from build123d import *

# Parameters (mm, degrees)
SKIZZE4_R                                   = 11.5
SCHNITT_LINEAR_AUSTRAGEN1_DEPTH             = 2.1
SCHNITT_LINEAR_START                        = -8
SKIZZE5_R                                   = 1
SCHNITT_LINEAR_AUSTRAGEN2_DEPTH             = 1
SCHNITT_LINEAR_AUSTRAGEN3_REACH             = 31.825
SCHNITT_LINEAR_AUSTRAGEN3_DIRECTION_2_DEPTH = 18.575
SKIZZE7_R                                   = 0.85
SCHNITT_LINEAR_AUSTRAGEN4_DEPTH             = 10


with BuildPart() as part:
    # Skizze3 → Rotation1 (revolve)
    with BuildSketch(Plane(origin=(0, 0, 0), x_dir=(0, 0, -1), z_dir=(1, 0, 0))):
        Polygon((-1.5, 4.2), (0, 4.2), (0, 0.5), (11, 0.5), (11, 4.2), (12.5, 4.2), (12.5, -12.875), (-1.5, -12.875), align=None)
    revolve(axis=Axis((0, -19.5, -13), (0, 0, 1)))

    # Skizze4 → Schnitt-Linear austragen1 (cut)
    with BuildSketch(Plane.XY.offset(1.5)):
        with Locations((0, -19.5)):
            Circle(SKIZZE4_R)
    extrude(amount=-SCHNITT_LINEAR_AUSTRAGEN1_DEPTH, mode=Mode.SUBTRACT)

    # Skizze5 → Schnitt-Linear austragen2 (cut)
    with BuildSketch(Plane.XY.offset(1.5).offset(SCHNITT_LINEAR_START)):
        with Locations((6.01040764, -13.48959236)):
            Circle(SKIZZE5_R)
        with Locations((7.573555456, -23.358919248)):
            Circle(SKIZZE5_R)
        with Locations((-1.329692953, -27.895350895)):
            Circle(SKIZZE5_R)
        with Locations((-8.395350895, -20.829692953)):
            Circle(SKIZZE5_R)
        with Locations((-3.858919248, -11.926444544)):
            Circle(SKIZZE5_R)
    extrude(amount=-SCHNITT_LINEAR_AUSTRAGEN2_DEPTH, mode=Mode.SUBTRACT)

    # Skizze6 → Schnitt-Linear austragen3 (cut, up to next)
    with BuildSketch(Plane(origin=(9.01325694, -13.375, -16.436641525), x_dir=(1, 0, 0), z_dir=(0, 1, 0)), mode=Mode.PRIVATE) as schnitt_linear_austragen3_sk1:
        with BuildLine():
            Line((-10.01325694, -4.836641525), (-8.01325694, -4.836641525))
            ThreePointArc((-8.01325694, -4.836641525), (-5.51325694, -7.336641525), (-8.01325694, -9.836641525))
            Line((-8.01325694, -9.836641525), (-10.01325694, -9.836641525))
            ThreePointArc((-10.01325694, -9.836641525), (-12.51325694, -7.336641525), (-10.01325694, -4.836641525))
        make_face()
    schnitt_linear_austragen3_tool1 = extrude(schnitt_linear_austragen3_sk1.sketch, amount=-SCHNITT_LINEAR_AUSTRAGEN3_REACH, mode=Mode.PRIVATE) & part.part
    add(schnitt_linear_austragen3_tool1.solids().sort_by_distance((0, -13.375, -9.1))[0], mode=Mode.SUBTRACT)
    add(schnitt_linear_austragen3_tool1.solids().sort_by_distance((0, -13.375, -9.1))[1], mode=Mode.SUBTRACT)

    # Skizze6 → Schnitt-Linear austragen3 direction 2 (cut)
    with BuildSketch(Plane(origin=(9.01325694, -13.375, -16.436641525), x_dir=(1, 0, 0), z_dir=(0, 1, 0))):
        with BuildLine():
            Line((-10.01325694, -4.836641525), (-8.01325694, -4.836641525))
            ThreePointArc((-8.01325694, -4.836641525), (-5.51325694, -7.336641525), (-8.01325694, -9.836641525))
            Line((-8.01325694, -9.836641525), (-10.01325694, -9.836641525))
            ThreePointArc((-10.01325694, -9.836641525), (-12.51325694, -7.336641525), (-10.01325694, -4.836641525))
        make_face()
    extrude(amount=SCHNITT_LINEAR_AUSTRAGEN3_DIRECTION_2_DEPTH, mode=Mode.SUBTRACT)

    # Skizze7 → Schnitt-Linear austragen4 (cut)
    with BuildSketch(Plane.XY.offset(1.5)):
        with Locations((-3.858919248, -11.926444544)):
            Circle(SKIZZE7_R)
        with Locations((6.01040764, -13.48959236)):
            Circle(SKIZZE7_R)
        with Locations((7.573555456, -23.358919248)):
            Circle(SKIZZE7_R)
        with Locations((-1.329692953, -27.895350895)):
            Circle(SKIZZE7_R)
        with Locations((-8.395350895, -20.829692953)):
            Circle(SKIZZE7_R)
    extrude(amount=-SCHNITT_LINEAR_AUSTRAGEN4_DEPTH, mode=Mode.SUBTRACT)


solid = part.part
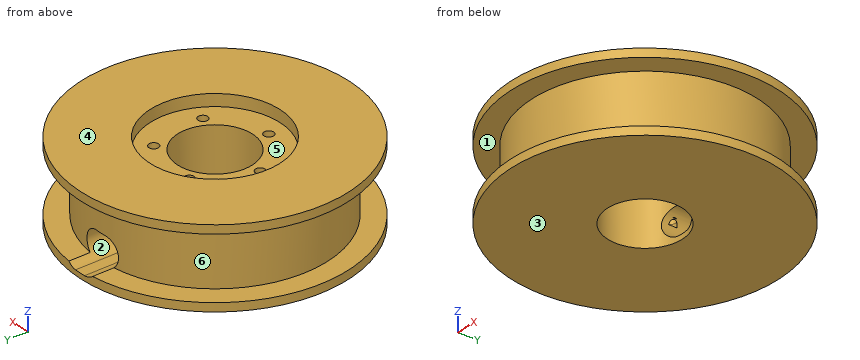
Source: CAD feature listing. Evaluate the final solid. Frame: model axes, mm. Face numbers are marked on the shaded views. A direction names the side the tool comes from. Round coordinates to 2 decimals unless told otherwise and drop trailing zeros. Order: outer loops, then holes, each group sorted by start corner. A loop starts at its lowest first (then second) coordinate and runs counter-clockwise, first axis right, second up. Notation, with made-up numbers: (89, 13.25) - (119, 13.25) arc R27 ccw to (119, 38.25) - close; hole circle Ø9 at (-3.75, -31.75). An arc over 180 degrees is marked (long way). Use a Markdown table: item, result. Add a question column.
1. First-contact query: pin 1 (2 mm diameter, centred on x = 7.5, y = -23.5, fed in from +Z); pin 2 (6 mm diameter, centred on x = -2.5, z = -9, fed in from +Y); pin 3 (3 mm diameter, centred on y = -1, z = 0, fed in from -X). Flat tips, straight axial feed; report the tip coordinate or a pass-through.
2. Section query B-B (z = -5). Return the cut outline in (x, y) (3 decimals).
3. Section query A-A (y = -9). Return the cut outline in (x, z).
4. Mould query, pull axis Y, two halves, no side actions, for the marked faces 4, 5 and 6. Classes: +Y half, -Y half, draft (parallel to the pull), parting line (faces both ways), or undercut.
5. Section query D-D (x = 18.5). Return the cut outline in (y, z), then the cut area to 3 significant figures.
6. Set-up query: the marked faces 1, 2 and 3. Return all of +Z, -Z, +X, -X, +Y, -Y with unobstructed straight access to the full face (end or side cutting, diameter ignored); none if empty.
7. Section query C-C (y = -17.5). Return the cut outline in (x, z), then the cut area to 3 significant figures.
8. Line query: probe 1 along Y at (x, z) = (0, -2) (3 decimals); probe 2 along X at (y, z) = (-24, -4); probe 3 along Z at (x, y) = (-21, -19.5). Output: solid intervals per line, ascending.
Derived:
| question | item | result |
|---|---|---|
| 1 | pin 1 | z = -0.6 |
| 1 | pin 2 | y = 4.18 |
| 1 | pin 3 | x = -16.51 |
| 2 | outline | circle Ø40 at (0, -19.5); hole circle Ø1.7 at (-8.395, -20.83); hole circle Ø13.25 at (0, -19.5); hole circle Ø1.7 at (-3.859, -11.926); hole circle Ø1.7 at (-1.33, -27.895); hole circle Ø1.7 at (6.01, -13.49); hole circle Ø1.7 at (7.574, -23.359) |
| 3 | outline | (-21.25, -12.5) - (21.25, -12.5) - (21.25, -11) - (17.02, -11) - (17.02, 0) - (21.25, 0) - (21.25, 1.5) - (4.69, 1.5) - (4.69, -0.6) - (-4.69, -0.6) - (-4.69, 1.5) - (-21.25, 1.5) - (-21.25, 0) - (-17.02, 0) - (-17.02, -11) - (-21.25, -11) - close; hole (-1, -11.6) - (1, -11.6) arc R2.5 ccw to (1, -6.6) - (-1, -6.6) arc R2.5 ccw to start |
| 4 | face 4 | draft |
| 4 | face 5 | undercut |
| 4 | face 6 | parting line |
| 5 | outline | (-34.31, -12.5) - (-4.69, -12.5) - (-4.69, -11) - (-11.9, -11) - (-11.9, 0) - (-4.69, 0) - (-4.69, 1.5) - (-34.31, 1.5) - (-34.31, 0) - (-27.1, 0) - (-27.1, -11) - (-34.31, -11) - close |
| 5 | area | 256 mm2 |
| 6 | face 1 | none |
| 6 | face 2 | +Y |
| 6 | face 3 | -Z, +X, -X, +Y, -Y |
| 7 | outline | (-23.62, -12.5) - (-6.32, -12.5) - (-6.32, -0.6) - (-11.32, -0.6) - (-11.32, 1.5) - (-23.62, 1.5) - (-23.62, 0) - (-19.9, 0) - (-19.9, -11) - (-23.62, -11) - close; (6.32, -12.5) - (23.62, -12.5) - (23.62, -11) - (19.9, -11) - (19.9, 0) - (23.62, 0) - (23.62, 1.5) - (11.32, 1.5) - (11.32, -0.6) - (6.32, -0.6) - close |
| 7 | area | 382 mm2 |
| 8 | probe 1 | -39.5 to -26.125, -12.875 to 0.5 |
| 8 | probe 2 | -19.49 to -4.86, 4.86 to 7.02, 8.13 to 19.49 |
| 8 | probe 3 | -12.5 to -11, 0 to 1.5 |
